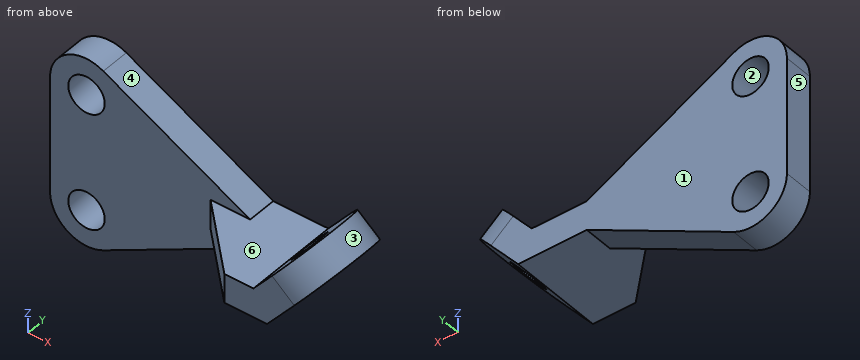
Autodesk Inventor part; units mm, degrees
ref_plane "YZ Plane" through (0, 0, 0) normal (1, 0, 0) x (0, 1, 0)
ref_plane "XZ Plane" through (0, 0, 0) normal (0, 1, 0) x (-1, 0, 0)
sketch "草图1" plane through (0, 0, 0) normal (0, 1, 0) x (-1, 0, 0)
  line L0 (55.5004, 0) -> (-70.183, 0)
  line L1 (21.9957, -8) -> (21.9957, 8)
  line L2 (14.6949, 12.4392) -> (-9.3051, 0)
  line L3 (14.6949, -12.4392) -> (-9.3051, 0)
  arc A0 (14.6949, -12.4392) -> (21.9957, -8) centre (16.9957, -8) ccw
  arc A1 (21.9957, 8) -> (14.6949, 12.4392) centre (16.9957, 8) ccw
  circle A2 centre (16.9957, -8) radius 2.5
  circle A3 centre (16.9957, 8) radius 2.5
  point P0 (0, 0)
  dimension "d0" = 5
  dimension "d1" = 16
  dimension "d2" = 24
  dimension "d3" = 5
  dimension "d4" = 5
extrude "拉伸1" add sketch "草图1" along normal blind 4
sketch "草图2" plane through (0, 0, 0) normal (0, 0, 1) x (1, 0, 0)
  line L0 (9.3051, 0) -> (-14.6949, 0)
  line L1 (9.3051, 0) -> (9.3051, 4)
  line L2 (-14.6949, 4) -> (9.3051, 4)
  line L3 (-14.6949, 0) -> (-14.6949, 4)
  line L4 (0, 4) -> (13, 4)
  line L5 (13, 4) -> (13, -9)
  line L6 (13, -9) -> (9, -9)
  line L7 (9, -9) -> (0, 0)
  line L8 (0, 0) -> (0, 4)
  dimension "d7" = 13
  dimension "d8" = 13
  dimension "d9" = 4
extrude "拉伸2" add sketch "草图2" along normal mid plane 4 contours L1 L4 L5 L6 L7 L0 | L0 L8 L2 L1
ref_plane "工作平面1" through (13, -9, 2) normal (0.7660444, 0, -0.6427876) x (0, 1, 0)
sketch "草图3" plane through (13, -9, 2) normal (0.7660444, 0, -0.6427876) x (0, 1, 0)
  line L0 (13, -3.0642) -> (13, 0)
  line L1 (0, 0) -> (13, 0)
  line L2 (0, -3.0642) -> (0, 0)
  line L3 (13, -3.0642) -> (0, -3.0642)
  line L4 (9, -7.9196) -> (9, -11.4204)
  line L5 (13, -7.9196) -> (9, -7.9196)
  line L6 (13, -7.9196) -> (13, -3.0642)
  line L7 (13, -3.0642) -> (0, -3.0642)
  line L8 (0, -3.0642) -> (0, -5.6353)
  line L9 (0, -5.6353) -> (9, -11.4204)
  line L10 (0, -3.0642) -> (13, -3.0642)
  line L11 (13, -3.0642) -> (13, 3.9358)
  line L12 (0, 3.9358) -> (0, -3.0642)
  arc A0 (13, 3.9358) -> (0, 3.9358) centre (6.5, 3.9358) ccw
  circle A1 centre (6.5, 3.9358) radius 2.5
  point P0 (9, -9.8883)
  dimension "d13" = 6.5
  dimension "d14" = 7
  dimension "d15" = 5
extrude "拉伸3" add sketch "草图3" along normal blind 4 contours L3 L2 L1 L0 | L1 L12 A0 L11
sketch "草图4" plane through (0, 4, 0) normal (0, 1, 0) x (1, 0, 0)
  line L0 (13, -2) -> (5.4463, -2)
  line L1 (14.0946, 2.9184) -> (18.5941, -2.4439)
  line L2 (13, 2) -> (14.0946, 2.9184)
  line L3 (13, 2) -> (14.8652, 2)
  point P0 (0, 0)
extrude "拉伸4" cut sketch "草图4" against normal blind 20
Could you check a few things on this model? Use its own coordinates, in mm. Face numbers are marked on the shaded views. A direction names the side the tool comes from. Give positions to 0.01 mm unless a question says otherwise; leave off trailing zeros. Order: outer loops, then holes, each group sorted by start corner. A loop starts at its lowest first (then second) coordinate and runs counter-clockwise, first axis right, second up.
Q1. We'd pull the mould along Z, two halves only. Please class the marked faces 1, 2 and 3: +Z half, -Z half, draft (parallel to the pull), parting line (faces both ways), or undercut.
Q2. If I drill on line 1 along X through (y, z) = (2.5, 7.5); line 2 along X through (y, z) = (2.25, 7.25); line 3 along Y through (x, z) = (-0.5, 4.75), over which ranges is the centre line in solid material (lowest first)?
Q3. Suppose I cut it at D-D, the plane z = -0.5. Write out the boundary of the cut face in (x, y), and give its area (3 significant figures).
Q4. Suppose I cut it at C-C, the plane x = 4.5. Write out the boundary of the cut face in (y, z).
Q5. For the marked faces 4, 5 and 6, which set-ups out of +Z, -Z, +X, -X, +Y, -Y let a thin tool reach every point of the face, with its end or its side?
Q6. I'm going to push flat-ended pins straight in: P1, Ø10, axis at x = 5.5, z = -8, coming from the +Y side; P2, Ø2, axis at y = 1, z = 9.5, coming from the +X side; P3, Ø2, axis at x = 17.5, y = -3, coming from the -Z side; P4, Ø13, axis at x = -5, z = -1.5, coming from the -Y side. Where does each tip first touch, or does it pass through?
Q7. Suppose I cut it at A-A, the plane y = 2.75. Write out the boundary of the cut face in (x, z).
Q8. Suppose I cut it at B-B, the plane y = -1.75. Write out the boundary of the cut face in (x, z), and give its area (3 significant figures).
Solution:
1. face 1: draft
1. face 2: undercut
1. face 3: +Z half
2. line 1: x = -22 to -19.45, -14.55 to -5.17, 17.62 to 19.03
2. line 2: x = -22 to -19.38, -14.61 to -4.68, 17.41 to 19.77
2. line 3: y = 0 to 4
3. outline: (-22, 0) - (0, 0) - (9, -9) - (16.12, -9) - (16.12, 4) - (-22, 4) - close
3. area: 257 mm2
4. outline: (-4.5, -2) - (0, -2) - (0, -2.49) - (4, -2.49) - (4, 2.49) - (0, 2.49) - (0, 2) - (-4.5, 2) - close
5. face 4: +Z, +Y, -Y
5. face 5: +Z, -Z, -X, +Y, -Y
5. face 6: +Z, -Y
6. P1: passes through
6. P2: stops at x = 20.19
6. P3: stops at z = -0.05
6. P4: stops at y = -1.5
7. outline: (-22, -8) arc R5 ccw to (-14.69, -12.44) - (5.45, -2) - (14.87, -2) - (21.06, 5.38) - (17.99, 7.95) - (13, 2) - (5.45, 2) - (-14.69, 12.44) arc R5 ccw to (-22, 8) - close; hole circle Ø5 at (-17, -8); hole circle Ø5 at (-17, 8)
8. outline: (1.75, -2) - (14.87, -2) - (17.06, 0.62) - (14, 3.19) - (13, 2) - (1.75, 2) - close; (17.06, 6.84) - (20.13, 4.27) - (22.74, 7.39) - (19.68, 9.96) - close
8. area: 75.0 mm2
